from build123d import *

# Parameters (mm, degrees)
F1_DEPTH = 101.6
F2_T     = -2.54


with BuildPart() as f1:
    # F0 (on Right) → F1 (new body)
    with BuildSketch(Plane.YZ):
        Polygon((53.1090894751, 316.3454540171), (80.8181880827, 360.9878815302), (53.1090894751, 367.1454756031), (14.6242498083, 316.3454540171), align=None)
        Polygon((31.5575774684, 273.2424150596), (53.1090894751, 316.3454540171), (14.6242498083, 316.3454540171), (0, 273.2424150596), align=None)
        Polygon((14.6242498083, 210.1272850298), (31.5575774684, 273.2424150596), (0, 273.2424150596), (-20.4879219231, 210.1272850298), align=None)
        Polygon((0, 125.4606056329), (14.6242498083, 210.1272850298), (-20.4879219231, 210.1272850298), (-36.1757530975, 119.3030314855), align=None)
        Polygon((0, 30.0181814408), (0, 125.4606056329), (-36.1757530975, 119.3030314855), (-36.1757530975, 0), align=None)
        Polygon((31.5575774684, -105.4484846724), (0, 30.0181814408), (-36.1757530975, 0), (0, -122.3818185592), align=None)
        Polygon((53.1090894751, -210.1272850298), (31.5575774684, -105.4484846724), (0, -122.3818185592), (14.6242498083, -211.6666735853), align=None)
        Polygon((53.1090894751, -248.6121184698), (53.1090894751, -210.1272850298), (14.6242498083, -211.6666735853), (14.6242498083, -248.6121184698), align=None)
    extrude(amount=F1_DEPTH)

    # F2
    f2_openings = [f1.faces().sort_by_distance(p)[0] for p in [
        (50.8, 66.963639, 364.066679),
        (50.8, 33.86667, -248.612118),
    ]]
    offset(amount=F2_T, openings=f2_openings, kind=Kind.INTERSECTION)


solid = f1.part
CAD build for the part. Positions are in the model's coordinates, mm. A direction names the side the tool comes from. Give positions to 0.01 mm unless a question says otherwise; leave off trailing zeros. Write each loop counter-clockwise with the first axis right and the second up, starting at its lowest first coordinate (ties: lowest second). Pieces come first, ordered by that corner, then holes. Notation, with made-up numbers: (85.25, -9) - (89.25, -9) arc R26 cw to (89.25, 22) - close; hole circle Ø6 at (71.5, 24). An arc over 180 degrees is marked (long way). Put each result on its own line as item: value.
(1) Tool access for faces 1 (the flat face through (50.09, 16, -38.66)), 2 (the flat face through (50, 50.569, -230)), 3 (the flat face through (50.12, -7.66, 241.42)): list every direction of +Z, -Z, +X, -X, +Y, -Y with a clear straight run to the whole face (end or side of a thin tool).
Working result:
face 1: +X, -X, +Y
face 2: -Z
face 3: none
(2) Pull direction Z, two halves, no side cores. Call faces 4 (the flat face through (50.12, 9.72, -166.01)), 5 (the flat face through (50.089, -18.341, -60.334)), 6 (the flat face through (50.089, 7.414, 295.096)): released by +Z, released by -Z, zero draft, split by the parting line, or undercut.
Working result:
face 4: undercut
face 5: released by -Z
face 6: released by +Z
(3) Saw through at A-A (z = 62). List the corners of the cut face in (x, y), then the cut area to 3 significant figures.
Working result:
outline: (0, -36.18) - (101.6, -36.18) - (101.6, 0) - (0, 0) - close; hole (2.54, -33.64) - (99.06, -33.64) - (99.06, -2.54) - (2.54, -2.54) - close
area: 674 mm^2
(4) Drop flat-ended pins along their axis: pin 1 Ø1 at (x, z) = (64, 262.5) entering from +Y; pin 2 Ø1 at (x, z) = (76.5, 246.5) entering from +Y; pin 3 Ø6 at (x, y) = (44, 17) entering from +Z. Give the stop position or say it passes through.
Working result:
pin 1: y = 28.81
pin 2: y = 24.52
pin 3: z = 323.44
(5) Saw through at C-C (z = -186.5). List the corners of the cut face in (x, y), then the cut area to 3 significant figures.
Working result:
outline: (0, 10.5) - (101.6, 10.5) - (101.6, 48.24) - (0, 48.24) - close; hole (2.54, 13.08) - (99.06, 13.08) - (99.06, 45.65) - (2.54, 45.65) - close
area: 690 mm^2
(6) Wall check: L1, parallel to Y at x = 33, z = 83; L2, parallel to X at y = -26.5, z = 46; L3, parallel to Y at x = 6.5, z = -217.5. Give the ranges that are in metal, low to high.
Working result:
L1: -36.18 to -33.64, -2.54 to 0
L2: 0 to 2.54, 99.06 to 101.6
L3: 14.62 to 17.16, 50.57 to 53.11
(7) Saw through at B-B (y = 67). List the corners of the cut face in (x, z), then the cut area to 3 significant figures.
Working result:
outline: (0, 338.73) - (101.6, 338.73) - (101.6, 364.06) - (99.06, 364.06) - (99.06, 343.54) - (2.54, 343.54) - (2.54, 364.06) - (0, 364.06) - close
area: 594 mm^2
